CAD build for the part. Positions are in the model's coordinates, mm. A direction names the side the tool comes from. Give positions to 0.01 mm unless a question says otherwise; leave off trailing zeros. Order: outer loops, then holes, each group sorted by start corner. A loop starts at its lowest first (then second) coordinate and runs counter-clockwise, first axis right, second up. Notation, with made-up numbers: M 23,23 L 58,23 A26 cw 58,56 Z; hole C 53.5,-7 d8. An arc over 180 degrees is marked long. Put each result on its own line as item: value. Start each with the question number.
1) Cut at C-C (x = 32). Write the cut outline in (y, z).
2) Tool access for faces 4 (the face through (5, 5, 16.706)), 5 (the face through (5.42, 12.86, 9.98)), 6 (the face through (12, 6, 15)): list every direction of +Z, -Z, +X, -X, +Y, -Y with a clear straight run to the whole face (end or side of a thin tool).
3) Two-plate mould, pull along Y, no slides. Class faces 1 (the face through (29.46, 24.08, 13.44)), 2 (the face through (31, 18, 10)), 3 (the face through (5.42, 13.45, 4.73)): released by +Y, released by -Y, zero draft, split by the parting line, or undercut.
4) Cut at D-D (y = 24.5). Write the cut outline in (x, z).
5) Cut at A-A (x = 18). Write the cut outline in (y, z), and give its area (3 significant figures).
6) Pin check, flat tips, straight feed: pin 1 (4.5 mm diameter, centred on x = 18, z = 19, fed in from -Y); pin 2 (3.5 mm diameter, centred on x = 3, z = 18, fed in from +Y); pin 3 (1.5 mm diameter, centred on y = 19, z = 8.5, fed in from -X). Stop position of each tip, or through.
7) Cut at B-B (y = 16.25). Write the cut outline in (x, z), and give its area (3 significant figures).
8) Drill centre lines: line 1 (Z direction, x = 18, y = 16.25); line 2 (Z direction, x = 30, y = 21); line 3 (X direction, y = 14, z = 11). Where is each one in solid material? Low to high. Write a range as [from, to].
```python
from build123d import *

# Parameters (mm, degrees)
SKETCH_1_W                   = 20
SKETCH_1_H                   = 40
EXTRUDE_1_DEPTH              = 30
CUT_EXTRUDE_1_DEPTH          = 11
SKETCH_13_W                  = 20
SKETCH_13_H                  = 30
CUT_EXTRUDE_5_DEPTH          = 10
SKETCH_14_W                  = 30
SKETCH_14_H                  = 30
EXTRUDE_5_DEPTH              = 20
HOLE_WIZARD_M2_1_D           = 2.4
HOLE_WIZARD_M2_1_CSINK_D     = 2.45
HOLE_WIZARD_M2_1_CSINK_ANGLE = 90
SKETCH_19_R                  = 2.5
CUT_EXTRUDE_6_DEPTH          = 12
SKETCH_20_W                  = 4
SKETCH_20_H                  = 30
CUT_EXTRUDE_7_DEPTH          = 49
SKETCH_22_W                  = 28
SKETCH_22_H                  = 22
CUT_EXTRUDE_8_DEPTH          = 10
SKETCH_23_W                  = 12
SKETCH_23_H                  = 3
CUT_EXTRUDE_9_DEPTH          = 23
SKETCH_24_W                  = 3.41182091
SKETCH_24_H                  = 4.86270688
CUT_EXTRUDE_10_DEPTH         = 11
SKETCH_25_W                  = 15
SKETCH_25_H                  = 22
CUT_EXTRUDE_11_DEPTH         = 12
FILLET_1_R                   = 3


with BuildPart() as part:
    # 草图1 → 凸台-拉伸1 (new body)
    with BuildSketch(Plane.XY):
        with Locations((10, 20)):
            Rectangle(SKETCH_1_W, SKETCH_1_H)
    extrude(amount=EXTRUDE_1_DEPTH)

    # 草图3 → 切除-拉伸1 (cut)
    with BuildSketch(Plane.ZY):
        with BuildLine():
            Line((2.42076783, 14.560970744), (2.46639251, 14.857401496))
            ThreePointArc((2.46639251, 14.857401496), (2.019622743, 14.921117547), (1.571223609, 14.972119278))
            Line((1.571223609, 14.972119278), (1.540625063, 14.673762896))
            ThreePointArc((1.540625063, 14.673762896), (0.958467816, 14.180991438), (0.443670306, 14.743765188))
            Line((0.443670306, 14.743765188), (0.451244703, 15.043586442))
            ThreePointArc((0.451244703, 15.043586442), (0.225645108, 15.048393221), (0, 15.049995588))
            Line((0, 15.049995588), (0, 16.111542732))
            ThreePointArc((0, 16.111542732), (8.761075107, 13.671748208), (15, 7.054736002))
            ThreePointArc((15, 7.054736002), (21.238924893, 13.671748208), (30, 16.111542732))
            Line((30, 16.111542732), (30, 15.049995588))
            ThreePointArc((30, 15.049995588), (29.774354892, 15.048393221), (29.548755297, 15.043586442))
            Line((29.548755297, 15.043586442), (29.556329694, 14.743765188))
            ThreePointArc((29.556329694, 14.743765188), (29.041532184, 14.180991438), (28.459374937, 14.673762896))
            Line((28.459374937, 14.673762896), (28.428776391, 14.972119278))
            ThreePointArc((28.428776391, 14.972119278), (27.980377257, 14.921117547), (27.53360749, 14.857401496))
            Line((27.53360749, 14.857401496), (27.57923217, 14.560970744))
            ThreePointArc((27.57923217, 14.560970744), (27.140146166, 13.937324811), (26.500073756, 14.352099545))
            Line((26.500073756, 14.352099545), (26.431798568, 14.644146289))
            ThreePointArc((26.431798568, 14.644146289), (25.993519676, 14.536561099), (25.558473085, 14.416571838))
            Line((25.558473085, 14.416571838), (25.641407746, 14.128345115))
            ThreePointArc((25.641407746, 14.128345115), (25.285156719, 13.453944659), (24.597553302, 13.78399361))
            Line((24.597553302, 13.78399361), (24.492709128, 14.064992722))
            ThreePointArc((24.492709128, 14.064992722), (24.071660856, 13.902569472), (23.655395377, 13.728253635))
            Line((23.655395377, 13.728253635), (23.774294539, 13.45290696))
            ThreePointArc((23.774294539, 13.45290696), (23.506658094, 12.738693055), (22.78267894, 12.978661705))
            Line((22.78267894, 12.978661705), (22.642966709, 13.244054422))
            ThreePointArc((22.642966709, 13.244054422), (22.245979893, 13.029428171), (21.855248772, 12.803613755))
            Line((21.855248772, 12.803613755), (22.008183484, 12.545614189))
            ThreePointArc((22.008183484, 12.545614189), (21.833503597, 11.803173817), (21.084894113, 11.949169057))
            Line((21.084894113, 11.949169057), (20.912580434, 12.194649806))
            ThreePointArc((20.912580434, 12.194649806), (20.546095554, 11.931302521), (20.187237779, 11.657653005))
            Line((20.187237779, 11.657653005), (20.37172692, 11.421186181))
            ThreePointArc((20.37172692, 11.421186181), (20.292837493, 10.662564255), (19.531742677, 10.712217544))
            Line((19.531742677, 10.712217544), (19.329623065, 10.93380379))
            ThreePointArc((19.329623065, 10.93380379), (18.999585753, 10.626007863), (18.678423221, 10.308962775))
            Line((18.678423221, 10.308962775), (18.891473749, 10.097864989))
            ThreePointArc((18.891473749, 10.097864989), (18.909654637, 9.335368941), (18.148422038, 9.287874734))
            Line((18.148422038, 9.287874734), (17.919775562, 9.481971593))
            ThreePointArc((17.919775562, 9.481971593), (17.631540148, 9.134720523), (17.35328321, 8.779423413))
            Line((17.35328321, 8.779423413), (17.591438718, 8.597119392))
            ThreePointArc((17.591438718, 8.597119392), (17.706394965, 7.843119504), (16.957374371, 7.699248319))
            Line((16.957374371, 7.699248319), (16.705910455, 7.86270688))
            ThreePointArc((16.705910455, 7.86270688), (16.4641531, 7.481634261), (16.233316031, 7.093849259))
            Line((16.233316031, 7.093849259), (16.492712825, 6.943296595))
            ThreePointArc((16.492712825, 6.943296595), (16.68180457, 6.174165972), (15.906222101, 6.013575078))
            Line((15.906222101, 6.013575078), (15.906222101, 3.404183419))
            Line((15.906222101, 3.404183419), (14.093777899, 3.404183419))
            Line((14.093777899, 3.404183419), (14.093777899, 6.013575078))
            ThreePointArc((14.093777899, 6.013575078), (13.31819543, 6.174165972), (13.507287175, 6.943296595))
            Line((13.507287175, 6.943296595), (13.766683969, 7.093849259))
            ThreePointArc((13.766683969, 7.093849259), (13.5358469, 7.481634261), (13.294089545, 7.86270688))
            Line((13.294089545, 7.86270688), (13.042625629, 7.699248319))
            ThreePointArc((13.042625629, 7.699248319), (12.293605035, 7.843119504), (12.408561282, 8.597119392))
            Line((12.408561282, 8.597119392), (12.64671679, 8.779423413))
            ThreePointArc((12.64671679, 8.779423413), (12.368459852, 9.134720523), (12.080224438, 9.481971593))
            Line((12.080224438, 9.481971593), (11.851577962, 9.287874734))
            ThreePointArc((11.851577962, 9.287874734), (11.090345363, 9.335368941), (11.108526251, 10.097864989))
            Line((11.108526251, 10.097864989), (11.321576779, 10.308962775))
            ThreePointArc((11.321576779, 10.308962775), (11.000414247, 10.626007863), (10.670376935, 10.93380379))
            Line((10.670376935, 10.93380379), (10.468257323, 10.712217544))
            ThreePointArc((10.468257323, 10.712217544), (9.707162507, 10.662564255), (9.62827308, 11.421186181))
            Line((9.62827308, 11.421186181), (9.812762221, 11.657653005))
            ThreePointArc((9.812762221, 11.657653005), (9.453904446, 11.931302521), (9.087419566, 12.194649806))
            Line((9.087419566, 12.194649806), (8.915105887, 11.949169057))
            ThreePointArc((8.915105887, 11.949169057), (8.166496403, 11.803173817), (7.991816516, 12.545614189))
            Line((7.991816516, 12.545614189), (8.144751228, 12.803613755))
            ThreePointArc((8.144751228, 12.803613755), (7.754020107, 13.029428171), (7.357033291, 13.244054422))
            Line((7.357033291, 13.244054422), (7.21732106, 12.978661705))
            ThreePointArc((7.21732106, 12.978661705), (6.493341906, 12.738693055), (6.225705461, 13.45290696))
            Line((6.225705461, 13.45290696), (6.344604623, 13.728253635))
            ThreePointArc((6.344604623, 13.728253635), (5.928339144, 13.902569472), (5.507290872, 14.064992722))
            Line((5.507290872, 14.064992722), (5.402446698, 13.78399361))
            ThreePointArc((5.402446698, 13.78399361), (4.714843281, 13.453944659), (4.358592254, 14.128345115))
            Line((4.358592254, 14.128345115), (4.441526915, 14.416571838))
            ThreePointArc((4.441526915, 14.416571838), (4.006480324, 14.536561099), (3.568201432, 14.644146289))
            Line((3.568201432, 14.644146289), (3.499926244, 14.352099545))
            ThreePointArc((3.499926244, 14.352099545), (2.859853834, 13.937324811), (2.42076783, 14.560970744))
        make_face()
    extrude(amount=-CUT_EXTRUDE_1_DEPTH, mode=Mode.SUBTRACT)

    # 草图13 → 切除-拉伸5 (cut)
    with BuildSketch(Plane(origin=(0, 40, 0), x_dir=(1, 0, 0), z_dir=(0, 1, 0))):
        with Locations((10, -15)):
            Rectangle(SKETCH_13_W, SKETCH_13_H)
    extrude(amount=-CUT_EXTRUDE_5_DEPTH, mode=Mode.SUBTRACT)

    # 草图14 → 凸台-拉伸5 (add)
    with BuildSketch(Plane(origin=(20, 0, 0), x_dir=(0, 0, -1), z_dir=(1, 0, 0))):
        with Locations((-15, 15)):
            Rectangle(SKETCH_14_W, SKETCH_14_H)
    extrude(amount=EXTRUDE_5_DEPTH)

    # M2 间隙孔1 (through all)
    with Locations(Plane(origin=(0, 30, 0), x_dir=(1, 0, 0), z_dir=(0, 1, 0))):
        with Locations((18, -11), (30, -11), (18, -19), (30, -19)):
            CounterSinkHole(HOLE_WIZARD_M2_1_D / 2, HOLE_WIZARD_M2_1_CSINK_D / 2, counter_sink_angle=HOLE_WIZARD_M2_1_CSINK_ANGLE)

    # 草图19 → 切除-拉伸6 (cut)
    with BuildSketch(Plane(origin=(0, 30, 0), x_dir=(1, 0, 0), z_dir=(0, 1, 0))):
        with Locations((18, -11)):
            Circle(SKETCH_19_R)
        with Locations((30, -11)):
            Circle(SKETCH_19_R)
        with Locations((30, -19)):
            Circle(SKETCH_19_R)
        with Locations((18, -19)):
            Circle(SKETCH_19_R)
    extrude(amount=-CUT_EXTRUDE_6_DEPTH, mode=Mode.SUBTRACT)

    # 草图20 → 切除-拉伸7 (cut)
    with BuildSketch(Plane(origin=(40, 0, 0), x_dir=(0, 0, -1), z_dir=(1, 0, 0))):
        with Locations((-28, 15)):
            Rectangle(SKETCH_20_W, SKETCH_20_H)
        with Locations((-2, 15)):
            Rectangle(SKETCH_20_W, SKETCH_20_H)
    extrude(amount=-CUT_EXTRUDE_7_DEPTH, mode=Mode.SUBTRACT)

    # 草图22 → 切除-拉伸8 (cut)
    with BuildSketch(Plane.XZ):
        with Locations((26, 15)):
            Rectangle(SKETCH_22_W, SKETCH_22_H)
    extrude(amount=-CUT_EXTRUDE_8_DEPTH, mode=Mode.SUBTRACT)

    # 草图23 → 切除-拉伸9 (cut, through all)
    with BuildSketch(Plane.XY.offset(26)):
        with Locations((6, 1.5)):
            Rectangle(SKETCH_23_W, SKETCH_23_H)
    extrude(amount=-CUT_EXTRUDE_9_DEPTH, mode=Mode.SUBTRACT)

    # 草图24 → 切除-拉伸10 (cut)
    with BuildSketch(Plane.ZY):
        with Locations((15, 5.43135344)):
            Rectangle(SKETCH_24_W, SKETCH_24_H)
    extrude(amount=-CUT_EXTRUDE_10_DEPTH, mode=Mode.SUBTRACT)

    # 草图25 → 切除-拉伸11 (cut)
    with BuildSketch(Plane(origin=(0, 30, 0), x_dir=(1, 0, 0), z_dir=(0, 1, 0))):
        with Locations((7.5, -15)):
            Rectangle(SKETCH_25_W, SKETCH_25_H)
    extrude(amount=-CUT_EXTRUDE_11_DEPTH, mode=Mode.SUBTRACT)

    # 圆角1
    fillet_1_edges = [part.edges().sort_by_distance(p)[0] for p in [
        (15, 18, 15),
    ]]
    fillet(fillet_1_edges, radius=FILLET_1_R)


solid = part.part
```
Solution:
1. outline: M 10,4 L 30,4 L 30,9.5 L 18,9.5 L 18,12.5 L 30,12.5 L 30,17.5 L 18,17.5 L 18,20.5 L 30,20.5 L 30,26 L 10,26 Z
2. face 4: -X, -Y
2. face 5: -X
2. face 6: +Z, -Z, +X, -Y
3. face 1: zero draft
3. face 2: released by +Y
3. face 3: undercut
4. outline: M 15,4 L 40,4 L 40,26 L 15,26 Z; hole C 18,11 d5; hole C 18,19 d5; hole C 30,11 d5; hole C 30,19 d5
5. outline: M 10,4 L 30,4 L 30,8.5 L 18,8.5 L 18,9.8 L 10,9.8 Z; M 10,12.2 L 18,12.2 L 18,13.5 L 30,13.5 L 30,16.5 L 18,16.5 L 18,17.8 L 10,17.8 Z; M 10,20.2 L 18,20.2 L 18,21.5 L 30,21.5 L 30,26 L 10,26 Z
5. area: 282 mm²
6. pin 1: y = 10
6. pin 2: y = 18
6. pin 3: x = 13.2
7. outline: M 0,4 L 40,4 L 40,26 L 0,26 Z; hole C 18,11 d2.4; hole C 18,19 d2.4; hole C 30,11 d2.4; hole C 30,19 d2.4
7. area: 862 mm²
8. line 1: [4, 9.8], [12.2, 17.8], [20.2, 26]
8. line 2: [4, 8.5], [13.5, 16.5], [21.5, 26]
8. line 3: [0, 16.8], [19.2, 28.8], [31.2, 40]
